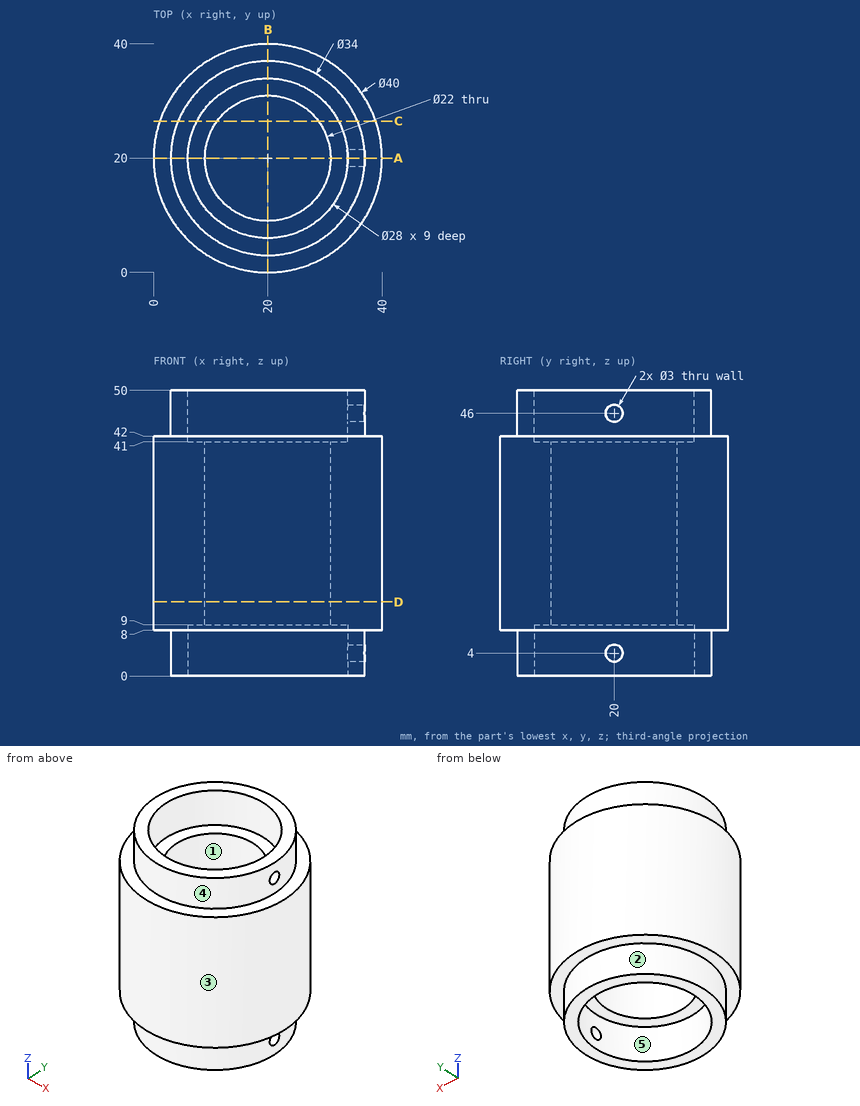
Can you work these out from the drawing? Everything is in mm from the part's minimum corner. A direction names the side the tool comes from. Give positions to 0.01 mm unless a question says otherwise; leave off trailing zeros. Order: outer loops, then holes, each group sorted by start corner. A loop starts at its lowest first (then second) coordinate and runs counter-clockwise, first axis right, second up. Notation, with made-up numbers: M 45.25,15 L 63.25,15 A32 cw 63.25,44 Z; hole C -13,-13.75 d10. An arc over 180 degrees is marked long. Use a Markdown table: item, result. Add a question column.
Item 1: Suppose I cut it at C-C (y = 26.5). List the corners of the cut face in (x, z) for me.
Item 2: Will these pins go through, and if not, where does the flat tip stop? pin 1 (4 mm diameter, centred on x = 35, y = 34.5, fed in from -Z); pin 2 (1.8 mm diameter, centred on y = 20, z = 46, fed in from +X); pin 3 (5 mm diameter, centred on x = 15.5, z = 21, fed in from +Y).
Item 3: We'd pull the mould along Y, two halves only. Please class the marked faces 1 and 2: +Y half, -Y half, draft (parallel to the pull), parting line (faces both ways), or undercut.
Item 4: Suppose I cut it at A-A (y = 20). Count the separate pieces of the cut face and the enclosed holes in it, then the cut area to 3 significant figures.
Item 5: For the marked faces 3, 4 and 5, which set-ups out of +Z, -Z, +X, -X, +Y, -Y let a thin tool reach every point of the face, with its end or its side?
Item 6: Suppose I cut it at B-B (x = 20). List the corners of the cut face in (y, z) for me, then the cut area to 3 significant figures.
Item 7: Suppose I cut it at D-D (z = 13). List the corners of the cut face in (x, y) for me.
Item 8: If I drill on L1, parallel to Y at x = 20, z = 34; L2, parallel to Z at x = 36, y = 20; L3, parallel to Y at x = 20, z = 3.25, over which ranges is the centre line in solid material (lowest first)? Write a range as [from, to].
Answer sheet:
| question | item | result |
|---|---|---|
| 1 | outline | M 1.09,8 L 4.29,8 L 4.29,0 L 7.6,0 L 7.6,9 L 11.13,9 L 11.13,41 L 7.6,41 L 7.6,50 L 4.29,50 L 4.29,42 L 1.09,42 Z; M 28.87,9 L 32.4,9 L 32.4,0 L 35.71,0 L 35.71,8 L 38.91,8 L 38.91,42 L 35.71,42 L 35.71,50 L 32.4,50 L 32.4,41 L 28.87,41 Z |
| 2 | pin 1 | stops at z = 8 |
| 2 | pin 2 | stops at x = 6.03 |
| 2 | pin 3 | stops at y = 39.9 |
| 3 | face 1 | undercut |
| 3 | face 2 | parting line |
| 4 | separate pieces | 4 |
| 4 | enclosed holes | 0 |
| 4 | area | 678 mm² |
| 5 | face 3 | +Z, -Z |
| 5 | face 4 | +Z |
| 5 | face 5 | -Z |
| 6 | outline | M 0,8 L 3,8 L 3,0 L 6,0 L 6,9 L 9,9 L 9,41 L 6,41 L 6,50 L 3,50 L 3,42 L 0,42 Z; M 31,9 L 34,9 L 34,0 L 37,0 L 37,8 L 40,8 L 40,42 L 37,42 L 37,50 L 34,50 L 34,41 L 31,41 Z |
| 6 | area | 696 mm² |
| 7 | outline | C 20,20 d40; hole C 20,20 d22 |
| 8 | L1 | y = [0, 9], [31, 40] |
| 8 | L2 | z = [0, 2.5], [5.5, 44.5], [47.5, 50] |
| 8 | L3 | y = [3, 6], [34, 37] |
